```python
from build123d import *

# Parameters (mm, degrees)
ESQUISSE1_R        = 8
ESQUISSE1_R_2      = 6
BOSS_EXTRU_1_DEPTH = 4
CHANFREIN1_SIZE    = 0.2


with BuildPart() as part:
    # Esquisse1 → Boss.-Extru.1 (new body)
    with BuildSketch(Plane.XY):
        Circle(ESQUISSE1_R)
        Circle(ESQUISSE1_R_2, mode=Mode.SUBTRACT)
    extrude(amount=BOSS_EXTRU_1_DEPTH)

    # Chanfrein1
    chanfrein1_edges = [part.edges().sort_by_distance(p)[0] for p in [
        (-8, 0, 0),
        (-8, 0, 4),
        (-6, 0, 0),
        (-6, 0, 4),
    ]]
    chamfer(chanfrein1_edges, length=CHANFREIN1_SIZE)


solid = part.part
```
Part model, mm, in its own coordinate system. Round coordinates to 2 decimals unless told otherwise and drop trailing zeros. Loops run counter-clockwise (first coordinate to the right, second up) from the corner with the lowest first, then second, coordinate; pieces in that order, holes last. Notation, with made-up numbers: (88.25, -12) -> (123.25, -12) arc R16 ccw to (123.25, 4) -> close; hole circle Ø9 at (11.5, -38.5). An arc over 180 degrees is marked (long way). Use one line per item in the form item = value. Start each with the question number.
Item 1: Drop flat-ended pins along their axis: pin 1 Ø1.5 at (y, z) = (-0.5, 0.5) entering from -X; pin 2 Ø5 at (x, y) = (-3.5, 0.5) entering from +Z. Give the stop position or say it passes through.
Item 2: Band-saw the part on C-C (z = 2.95). List the corners of the cut face in (x, y), plus the area to 3 significant figures.
Item 3: Two-plate mould, pull along X, no slides. Class faces 1 (the flat face through (-3, -6, 4)), 2 (the cylindrical face through (-6, 0, 2)), 3 (the cylindrical face through (-1.73, -7.81, 1.97)): released by +X, released by -X, zero draft, split by the parting line, or undercut.
Item 4: Drill centre lines: line 1 along Y through (x, z) = (0, 1.15); line 2 along X through (y, z) = (5.5, 0.8); line 3 along Y through (x, z) = (2, 1.35). Where is each one in solid material? Low to high.
Item 5: Band-saw the part on A-A (x = 0). List the corners of the cut face in (y, z).
Data:
q1.pin_1 = -8
q1.pin_2 = 3.84
q2.outline = circle Ø16 at (0, 0); hole circle Ø12 at (0, 0)
q2.area = 88.0 mm^2
q3.face_1 = zero draft
q3.face_2 = undercut
q3.face_3 = split by the parting line
q4.line_1 = -8 to -6, 6 to 8
q4.line_2 = -5.81 to -2.4, 2.4 to 5.81
q4.line_3 = -7.75 to -5.66, 5.66 to 7.75
q5.outline = (-8, 0.2) -> (-7.8, 0) -> (-6.2, 0) -> (-6, 0.2) -> (-6, 3.8) -> (-6.2, 4) -> (-7.8, 4) -> (-8, 3.8) -> close; (6, 0.2) -> (6.2, 0) -> (7.8, 0) -> (8, 0.2) -> (8, 3.8) -> (7.8, 4) -> (6.2, 4) -> (6, 3.8) -> close
